```python
from build123d import *

# Parameters (mm, degrees)
SKETCH2_R           = 4.826
CUT_EXTRUDE1_DEPTH  = 25.4
SKETCH3_W           = 14.986
SKETCH3_H           = 14.986
BOSS_EXTRUDE1_DEPTH = 12.7


with BuildPart() as part:
    # Sketch1 → Revolve1 (revolve)
    with BuildSketch(Plane.XY):
        Polygon((12.7, 12.7), (12.7, 15.875), (152.4, 12.7), (152.4, 0), (12.7, 0), align=None)
    revolve(axis=Axis((12.7, 0, 0), (1, 0, 0)))

    # Sketch2 → Cut-Extrude1 (cut)
    with BuildSketch(Plane(origin=(152.4, 0, 0), x_dir=(0, 0, -1), z_dir=(1, 0, 0))):
        Circle(SKETCH2_R)
    extrude(amount=-CUT_EXTRUDE1_DEPTH, mode=Mode.SUBTRACT)

    # Sketch3 → Boss-Extrude1 (add)
    with BuildSketch(Plane.ZY.offset(-12.7)):
        Rectangle(SKETCH3_W, SKETCH3_H)
    extrude(amount=BOSS_EXTRUDE1_DEPTH)


solid = part.part
```
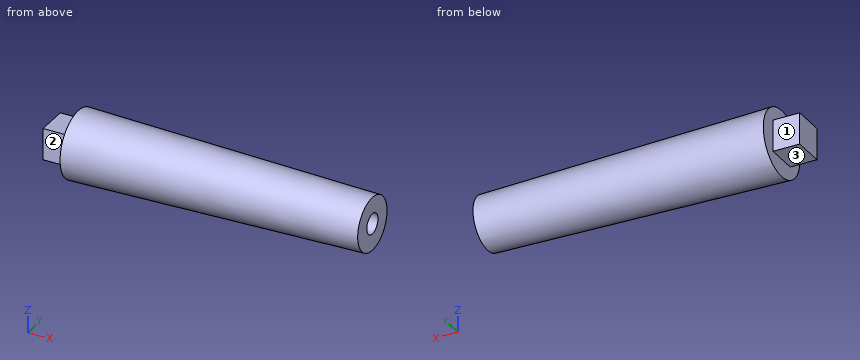
Build history of the part. All positions in model axes, mm. Face numbers are marked on the shaded views. A direction names the side the tool comes from. Give positions to 0.01 mm unless a question says otherwise; leave off trailing zeros. Loops run counter-clockwise (first coordinate to the right, second up) from the corner with the lowest first, then second, coordinate; pieces in that order, holes last.
1) Band-saw the part on A-A on z = 0. List the corners of the cut face in (x, y) (3 decimals), then the cut area to 3 significant figures.
Values follow:
outline: (0, -7.493) - (12.7, -7.493) - (12.7, -15.875) - (152.4, -12.7) - (152.4, -4.826) - (127, -4.826) - (127, 4.826) - (152.4, 4.826) - (152.4, 12.7) - (12.7, 15.875) - (12.7, 7.493) - (0, 7.493) - close
area: 3,940 mm2
2) Probe line 1 along Y through (x, z) = (147, 0); line 2 along Y through (x, z) = (136.25, 0); line 3 along X through (y, z) = (-4, 1.5). List the from-to ranges inside material, lowest first.
Values follow:
line 1: y = -12.82 to -4.83, 4.83 to 12.82
line 2: y = -13.07 to -4.83, 4.83 to 13.07
line 3: x = 0 to 127
3) 3-axis set-ups, long thin cutter, end or side, ignore diameter. For the marked faces 1, 2 and 3: which of +Z, -Z, +X, -X, +Y, -Y reach the whole face in a straight line?
Values follow:
face 1: +Z, -Z, -X, +Y
face 2: +Z, -Z, -X, -Y
face 3: -Z, -X, +Y, -Y
4) Drop flat-ended pins along their axis: P1, Ø14, axis at x = 6.5, z = -3.5, coming from the -Y side; P2, Ø3, axis at y = 0, z = -2.5, coming from the +X side; P3, Ø5, axis at x = 62.5, z = 6.5, coming from the -Y side; P4, Ø2, axis at y = 5.5, z = 12, coming from the +X side. Give the stop position or say it passes through.
Values follow:
P1: stops at y = -15.87
P2: stops at x = 127
P3: stops at y = -14.19
P4: stops at x = 152.4
5) Band-saw the part on B-B on x = 56.5. List the corners of the cut face in (y, z).
Values follow:
outline: circle Ø29.76 at (0, 0)
6) Band-saw the part on C-C on x = 119. List the corners of the cut face in (y, z), then the cut area to 3 significant figures.
Values follow:
outline: circle Ø26.92 at (0, 0)
area: 569 mm2
